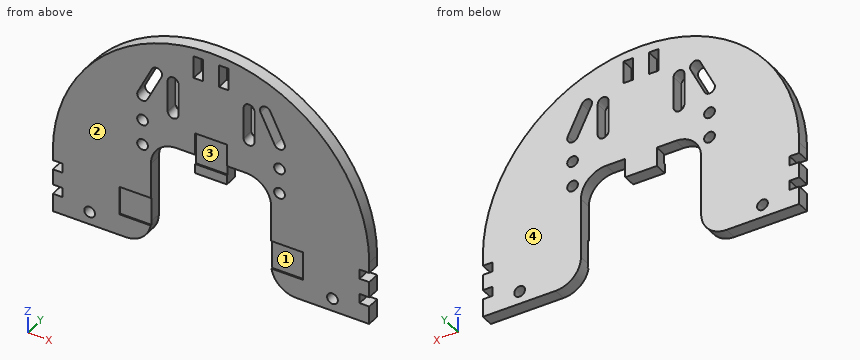
Autodesk Inventor part; units mm, degrees
ref_plane "YZ Plane" through (0, 0, 0) normal (1, 0, 0) x (0, 1, 0)
ref_plane "XZ Plane" through (0, 0, 0) normal (0, 1, 0) x (-1, 0, 0)
ref_plane "XY Plane" through (0, 0, 0) normal (0, 0, 1) x (1, 0, 0)
sketch "Эскиз1" plane through (0, 0, 0) normal (0, 1, 0) x (-1, 0, 0)
  line L0 (0, 0) -> (0, -235.2683) construction
  line L1 (250, -250) -> (250, -350)
  line L2 (250, -350) -> (135, -350)
  arc A0 (95, -310) -> (135, -350) centre (135, -310) ccw
  line L3 (95, -310) -> (95, -215)
  arc A1 (95, -215) -> (55, -175) centre (55, -215) ccw
  line L4 (25, -175) -> (25, -205)
  line L5 (25, -205) -> (0, -205)
  line L6 (55, -175) -> (25, -175)
  line L7 (60, -70) -> (60, -120) construction
  line L8 (51.5, -70) -> (51.5, -120)
  line L9 (68.5, -120) -> (68.5, -70)
  arc A2 (68.5, -70) -> (51.5, -70) centre (60, -70) ccw
  arc A3 (51.5, -120) -> (68.5, -120) centre (60, -120) ccw
  line L10 (85.9368, -64.05) -> (108.22, -108.81) construction
  line L11 (93.546, -60.2619) -> (115.8292, -105.0219)
  line L12 (100.6108, -112.5981) -> (78.3276, -67.8381)
  arc A4 (93.546, -60.2619) -> (78.3276, -67.8381) centre (85.9368, -64.05) ccw
  arc A5 (100.6108, -112.5981) -> (115.8292, -105.0219) centre (108.22, -108.81) ccw
  line L13 (12.5, -15) -> (27.43, -15)
  line L14 (27.43, -15) -> (27.43, -50.33)
  line L15 (27.43, -50.33) -> (12.5, -50.33)
  line L16 (12.5, -50.33) -> (12.5, -15)
  circle A6 centre (108.22, -148.81) radius 8.5
  circle A7 centre (108.22, -188.81) radius 8.5
  circle A8 centre (191.91, -330) radius 8.5
  line L17 (-250, -250) -> (-250, -350)
  line L18 (-250, -350) -> (-135, -350)
  arc A9 (-135, -350) -> (-95, -310) centre (-135, -310) ccw
  line L19 (-95, -310) -> (-95, -215)
  arc A10 (-55, -175) -> (-95, -215) centre (-55, -215) ccw
  line L20 (-25, -175) -> (-25, -205)
  line L21 (-25, -205) -> (0, -205)
  line L22 (-55, -175) -> (-25, -175)
  line L23 (-60, -70) -> (-60, -120) construction
  line L24 (-51.5, -70) -> (-51.5, -120)
  line L25 (-68.5, -120) -> (-68.5, -70)
  arc A11 (-51.5, -70) -> (-68.5, -70) centre (-60, -70) ccw
  arc A12 (-68.5, -120) -> (-51.5, -120) centre (-60, -120) ccw
  line L26 (-85.9368, -64.05) -> (-108.22, -108.81) construction
  line L27 (-93.546, -60.2619) -> (-115.8292, -105.0219)
  line L28 (-100.6108, -112.5981) -> (-78.3276, -67.8381)
  arc A13 (-78.3276, -67.8381) -> (-93.546, -60.2619) centre (-85.9368, -64.05) ccw
  arc A14 (-115.8292, -105.0219) -> (-100.6108, -112.5981) centre (-108.22, -108.81) ccw
  line L29 (-12.5, -15) -> (-27.43, -15)
  line L30 (-27.43, -15) -> (-27.43, -50.33)
  line L31 (-27.43, -50.33) -> (-12.5, -50.33)
  line L32 (-12.5, -50.33) -> (-12.5, -15)
  circle A15 centre (-108.22, -148.81) radius 8.5
  circle A16 centre (-108.22, -188.81) radius 8.5
  circle A17 centre (-191.91, -330) radius 8.5
  arc A18 (250, -250) -> (-250, -250) centre (0, -250) ccw
  line L33 (250, -321.45) -> (234.79, -321.45)
  line L34 (234.79, -321.45) -> (234.79, -306.5)
  line L35 (234.79, -306.5) -> (250, -306.5)
  line L36 (250, -281.62) -> (234.79, -281.62)
  line L37 (234.79, -281.62) -> (234.79, -266.67)
  line L38 (234.79, -266.67) -> (250, -266.67)
  line L39 (-250, -321.45) -> (-234.79, -321.45)
  line L40 (-234.79, -321.45) -> (-234.79, -306.5)
  line L41 (-234.79, -306.5) -> (-250, -306.5)
  line L42 (-250, -281.62) -> (-234.79, -281.62)
  line L43 (-234.79, -281.62) -> (-234.79, -266.67)
  line L44 (-234.79, -266.67) -> (-250, -266.67)
  point P0 (60, -95)
  point P1 (97.0784, -86.43)
  point P2 (-60, -95)
  point P3 (-97.0784, -86.43)
  dimension "d2" = 115
  dimension "d4" = 40
  dimension "d5" = 30
  dimension "d7" = 250
  dimension "d9" = 25
  dimension "d10" = 350
  dimension "d11" = 95
  dimension "d12" = 30
  dimension "d13" = 50
  dimension "d14" = 8.5
  dimension "d15" = 64.05
  dimension "d16" = 141.78
  dimension "d17" = 48.22
  dimension "d18" = 70
  dimension "d20" = 241.19
  dimension "d21" = 14.93
  dimension "d22" = 35.33
  dimension "d23" = 12.5
  dimension "d24" = 15
  dimension "d25" = 17
  dimension "d26" = 40
  dimension "d27" = 161.19
  dimension "d28" = 141.78
  dimension "d29" = 20
  dimension "d30" = 58.09
  dimension "d34" = 15.21
  dimension "d35" = 28.55
  dimension "d36" = 14.95
  dimension "d37" = 24.88
  dimension "d47" = 24.88
  dimension "d48" = 28.55
  dimension "d49" = 14.95
  dimension "d50" = 15.21
extrude "Пластина1" add sketch "Эскиз1" along normal blind 20 contours L1 L38 L37 L36 L35 L34 L33 L2 A0 L3 A1 L6 L4 L5 L21 L20 L22 A10 L19 A9 L18 L17 L39 L40 L41 L42 L43 L44 A18
sketch "Эскиз2" plane through (0, 0, 0) normal (0, -1, 0) x (1, 0, 0)
  arc A0 (100.6108, -112.5981) -> (115.8292, -105.0219) centre (108.22, -108.81) ccw
  line L0 (100.6108, -112.5981) -> (78.3276, -67.8381)
  arc A1 (93.546, -60.2619) -> (78.3276, -67.8381) centre (85.9368, -64.05) ccw
  line L1 (93.546, -60.2619) -> (115.8292, -105.0219)
  arc A2 (51.5, -120) -> (68.5, -120) centre (60, -120) ccw
  line L2 (51.5, -120) -> (51.5, -70)
  arc A3 (68.5, -70) -> (51.5, -70) centre (60, -70) ccw
  line L3 (68.5, -70) -> (68.5, -120)
  arc A4 (-115.8292, -105.0219) -> (-100.6108, -112.5981) centre (-108.22, -108.81) ccw
  line L4 (-115.8292, -105.0219) -> (-93.546, -60.2619)
  arc A5 (-78.3276, -67.8381) -> (-93.546, -60.2619) centre (-85.9368, -64.05) ccw
  line L5 (-78.3276, -67.8381) -> (-100.6108, -112.5981)
  arc A6 (-51.5, -70) -> (-68.5, -70) centre (-60, -70) ccw
  line L6 (-51.5, -70) -> (-51.5, -120)
  arc A7 (-68.5, -120) -> (-51.5, -120) centre (-60, -120) ccw
  line L7 (-68.5, -120) -> (-68.5, -70)
  line L8 (12.5, -15) -> (27.43, -15)
  line L9 (27.43, -15) -> (27.43, -50.33)
  line L10 (27.43, -50.33) -> (12.5, -50.33)
  line L11 (12.5, -50.33) -> (12.5, -15)
  line L12 (-27.43, -50.33) -> (-27.43, -15)
  line L13 (-27.43, -15) -> (-12.5, -15)
  line L14 (-12.5, -15) -> (-12.5, -50.33)
  line L15 (-12.5, -50.33) -> (-27.43, -50.33)
  circle A8 centre (191.91, -330) radius 8.5
  circle A9 centre (108.22, -188.81) radius 8.5
  circle A10 centre (108.22, -148.81) radius 8.5
  circle A11 centre (-191.91, -330) radius 8.5
  circle A12 centre (-108.22, -188.81) radius 8.5
  circle A13 centre (-108.22, -148.81) radius 8.5
  arc A14 (250, -250) -> (-250, -250) centre (0, -250) ccw
  line L16 (-250, -266.67) -> (-250, -250)
  line L17 (-234.79, -266.67) -> (-250, -266.67)
  line L18 (-234.79, -281.62) -> (-234.79, -266.67)
  line L19 (-250, -281.62) -> (-234.79, -281.62)
  line L20 (-250, -306.5) -> (-250, -281.62)
  line L21 (-234.79, -306.5) -> (-250, -306.5)
  line L22 (-234.79, -321.45) -> (-234.79, -306.5)
  line L23 (-250, -321.45) -> (-234.79, -321.45)
  line L24 (-250, -350) -> (-250, -321.45)
  line L25 (-135, -350) -> (-250, -350)
  arc A15 (-135, -350) -> (-95, -310) centre (-135, -310) ccw
  line L26 (-95, -215) -> (-95, -310)
  arc A16 (-55, -175) -> (-95, -215) centre (-55, -215) ccw
  line L27 (-25, -175) -> (-55, -175)
  line L28 (-25, -205) -> (-25, -175)
  line L29 (25, -205) -> (-25, -205)
  line L30 (25, -175) -> (25, -205)
  line L31 (55, -175) -> (25, -175)
  arc A17 (95, -215) -> (55, -175) centre (55, -215) ccw
  line L32 (95, -310) -> (95, -215)
  arc A18 (95, -310) -> (135, -350) centre (135, -310) ccw
  line L33 (250, -350) -> (135, -350)
  line L34 (250, -321.45) -> (250, -350)
  line L35 (25, -190) -> (-25, -190)
  line L36 (-25, -190) -> (-25, -140)
  line L37 (-25, -140) -> (25, -140)
  line L38 (25, -140) -> (25, -190)
  line L39 (95, -310) -> (95, -215)
  line L40 (95, -271.5) -> (145, -271.5)
  line L41 (145, -271.5) -> (145, -316.5)
  line L42 (145, -316.5) -> (95, -316.5)
  line L43 (95, -316.5) -> (95, -271.5)
  line L44 (-95, -215) -> (-95, -310)
  line L45 (-95, -316.5) -> (-145, -316.5)
  line L46 (-145, -316.5) -> (-145, -271.5)
  line L47 (-145, -271.5) -> (-95, -271.5)
  line L48 (-95, -271.5) -> (-95, -316.5)
  line L49 (234.79, -321.45) -> (250, -321.45)
  line L50 (234.79, -306.5) -> (234.79, -321.45)
  line L51 (250, -306.5) -> (234.79, -306.5)
  line L52 (250, -281.62) -> (250, -306.5)
  line L53 (234.79, -281.62) -> (250, -281.62)
  line L54 (234.79, -266.67) -> (234.79, -281.62)
  line L55 (250, -266.67) -> (234.79, -266.67)
  line L56 (250, -250) -> (250, -266.67)
  point P0 (0, 0)
  point P1 (0, -190)
  point P2 (0, -205)
  dimension "d38" = 50
  dimension "d39" = 45
  dimension "d40" = 33.5
  dimension "d41" = 50
  dimension "d42" = 50
  dimension "d43" = 50
  dimension "d44" = 15
extrude "Вырез1" cut sketch "Эскиз2" against normal blind 2 contours L42 L43 A18 | A18 L32 L40 L41 L42 | L45 L46 L47 L26 A15 | A15 L48 L45 | L30 L35 L28 L36 L37 L38
equation "\"d33\" = Толщина"
properties part number "Lift.03.00.00.02"
The listing builds one solid part. Answer for the finished solid, in the listing's coordinates (mm). Face numbers are marked on the shaded views. A direction names the side the tool comes from. Round coordinates to 2 decimals unless told otherwise and drop trailing zeros. Loops run counter-clockwise (first coordinate to the right, second up) from the corner with the lowest first, then second, coordinate; pieces in that order, holes last.
1) Consider line 1 (X direction, y = 11, z = -298); line 2 (X direction, y = 8.5, z = -82.5); line 3 (X direction, y = 11, z = -120.5). Determine where each line is inside the solid, lowest interval first.
Outcome:
line 1: x = -250 to -95, 95 to 250
line 2: x = -185.59 to -104.62, -85.63 to -68.5, -51.5 to 51.5, 68.5 to 85.63, 104.62 to 185.59
line 3: x = -213.85 to -68.49, -51.51 to 51.51, 68.49 to 213.85
2) For the marked faces 3 and 4, determine the directions among +Z, -Z, +X, -X, +Y, -Y from which every point of the face is accessible in a straight line to the end or side of a thin tool.
Outcome:
face 3: -Y
face 4: +Z, -Z, +X, -X, +Y
3) A cutting plane is placed at B-B on z = -148.81. Determine the outline of the cut face in (x, y).
Outcome:
outline: (-228.61, 0) - (-116.72, 0) - (-116.72, 20) - (-228.61, 20) - close; (-99.72, 0) - (-25, 0) - (-25, 2) - (25, 2) - (25, 0) - (99.72, 0) - (99.72, 20) - (-99.72, 20) - close; (116.72, 0) - (228.61, 0) - (228.61, 20) - (116.72, 20) - close
4) A cutting plane is placed at C-C on x = 0. Determine the outline of the cut face in (y, z), plus the area to 3 significant figures.
Outcome:
outline: (0, -205) - (20, -205) - (20, 0) - (0, 0) - (0, -140) - (2, -140) - (2, -190) - (0, -190) - close
area: 4,000 mm2
5) Given P1, Ø1.5, axis at y = 14, z = -72.5, coming from the +X side; P2, Ø6, axis at y = 10, z = -212.5, coming from the +X side; P3, Ø4, axis at y = 9, z = -61.5, coming from the -X side; P4, Ø13.5, axis at x = 108.22, z = -188.81, coming from the -Y side, each flat-ended and moving along its own axis, determine where each tip first touches the part or whether it passes through.
Outcome:
P1: stops at x = 176.8
P2: stops at x = 247.61
P3: stops at x = -166.49
P4: passes through
6) For a pull along Z with two mould halves and no side action, classify the marked faces 1 and 2 as released by +Z, released by -Z, zero draft, split by the parting line, or undercut.
Outcome:
face 1: undercut
face 2: zero draft
7) A cutting plane is placed at D-D on y = 16.5. Give the number of separate pieces and of enclosed holes in the cut face, plus the area to 3 significant figures.
Outcome:
separate pieces: 1
enclosed holes: 12
area: 109,000 mm2
8) A cutting plane is placed at A-A on x = 86. Determine the outline of the cut face in (y, z).
Outcome:
outline: (0, -189.72) - (20, -189.72) - (20, -83.25) - (0, -83.25) - close; (0, -55.55) - (20, -55.55) - (20, -15.26) - (0, -15.26) - close
